from build123d import *

# Parameters (mm, degrees)
SKETCH_1_R      = 17
SKETCH_1_R_2    = 10
EXTRUDE_1_DEPTH = 51
EXTRUDE_START   = -7
SKETCH_7_R      = 10
EXTRUDE_2_DEPTH = 10


with BuildPart() as part:
    # 草图1 → 凸台-拉伸1 (new body)
    with BuildSketch(Plane(origin=(0, 0, 0), x_dir=(1, 0, 0), z_dir=(0, 1, 0))):
        with Locations(Location((0, 0, 0), (0, 0, 270))):
            Circle(SKETCH_1_R)
        with Locations(Location((0, 0, 0), (0, 0, 270))):
            Circle(SKETCH_1_R_2, mode=Mode.SUBTRACT)
    extrude(amount=EXTRUDE_1_DEPTH)

    # 草图7 → 凸台-拉伸2 (add)
    with BuildSketch(Plane.XZ.offset(EXTRUDE_START)):
        with BuildLine():
            Line((-18, 22.737634002), (-18, -22.737634002))
            ThreePointArc((-18, -22.737634002), (0, -29), (18, -22.737634002))
            Line((18, -22.737634002), (18, 22.737634002))
            ThreePointArc((18, 22.737634002), (0, 29), (-18, 22.737634002))
        make_face()
        with Locations(Location((0, 0, 0), (0, 0, 90))):
            Circle(SKETCH_7_R, mode=Mode.SUBTRACT)
    extrude(amount=-EXTRUDE_2_DEPTH)


solid = part.part
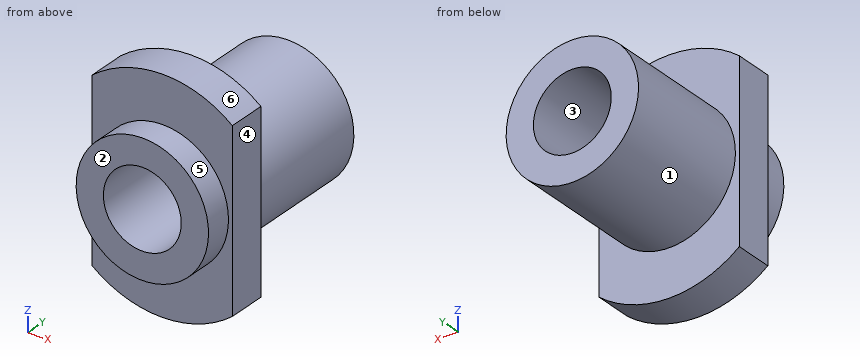
Geometry: final body of the model. Coordinates: model frame, mm. Face numbers are marked on the shaded views. A direction names the side the tool comes from. Round coordinates to 2 decimals unless told otherwise and drop trailing zeros. Order: outer loops, then holes, each group sorted by start corner. A loop starts at its lowest first (then second) coordinate and runs counter-clockwise, first axis right, second up. Notation, with made-up numbers: (-3, -6.75) -> (33, -6.75) arc R25 cw to (33, 13.25) -> close; hole circle Ø11 at (26, -35). An arc over 180 degrees is marked (long way). Put each result on its own line as item: value. Start each with the question number.
Q1. Line query: probe 1 along X at (y, z) = (33.5, 0); probe 2 along X at (y, z) = (11.5, 0); probe 3 along Y at (x, z) = (-16, -11). Output: solid intervals per line, ascending.
Q2. Reachability of the marked faces 5 and 6 from +Z, -Z, +X, -X, +Y, -Y: full face, straight path, thin tool, end or side. Return the list, or none.
Q3. Section C-C on y = 22. Return the cut outline in (x, z).
Q4. Section A-A on x = 0. Return the cut outline in (y, z), and give its area (3 significant figures).
Q5. Section B-B on z = 0. Return the cut outline in (x, y), and give its area (3 significant figures).
Q6. First-contact query: pin 1 (1 mm diameter, centred on x = -13.5, y = 35.5, fed in from -Z); pin 2 (1 mm diameter, centred on x = 5, z = 20.5, fed in from -Y); pin 3 (16 mm diameter, centred on x = 0, z = 0, fed in from -Y). Flat tips, straight axial feed; report the tip coordinate or a pass-through.
Q7. Section D-D on x = 15.5. Return the cut outline in (y, z), and give its area (3 significant figures).
Q8. Pull-direction query (X, two-part tool) for the marked faces 1, 2, 3 and 4; classes: +X half, -X half, draft (parallel to the pull), parting line (faces both ways), or undercut.
Ans:
1. probe 1: x = -17 to -10, 10 to 17
1. probe 2: x = -18 to -10, 10 to 18
1. probe 3: y = 7 to 17
2. face 5: -Y
2. face 6: +Z, +Y, -Y
3. outline: circle Ø34 at (0, 0); hole circle Ø20 at (0, 0)
4. outline: (0, -17) -> (7, -17) -> (7, -29) -> (17, -29) -> (17, -17) -> (51, -17) -> (51, -10) -> (0, -10) -> close; (0, 10) -> (51, 10) -> (51, 17) -> (17, 17) -> (17, 29) -> (7, 29) -> (7, 17) -> (0, 17) -> close
4. area: 954 mm2
5. outline: (-18, 7) -> (-17, 7) -> (-17, 0) -> (-10, 0) -> (-10, 51) -> (-17, 51) -> (-17, 17) -> (-18, 17) -> close; (10, 0) -> (17, 0) -> (17, 7) -> (18, 7) -> (18, 17) -> (17, 17) -> (17, 51) -> (10, 51) -> close
5. area: 734 mm2
6. pin 1: stops at z = -10.95
6. pin 2: stops at y = 7
6. pin 3: passes through
7. outline: (0, -6.98) -> (7, -6.98) -> (7, -24.51) -> (17, -24.51) -> (17, -6.98) -> (51, -6.98) -> (51, 6.98) -> (17, 6.98) -> (17, 24.51) -> (7, 24.51) -> (7, 6.98) -> (0, 6.98) -> close
7. area: 1,060 mm2
8. face 1: parting line
8. face 2: draft
8. face 3: undercut
8. face 4: +X half
